Source: three-view drawing plus pictorial views. Frame: mm from the lowest corner of the part. A direction names the side the tool comes from. Round coordinates to 2 decimals unless told otherwise and drop trailing zeros. Write each loop counter-clockwise with the first axis right and the second up, starting at its lowest first coordinate (ties: lowest second). Pieces come first, ordered by that corner, then holes. Notation, with made-up numbers: (70, 0) - (105, 0) arc R25 cw to (105, 35) - close; hole circle Ø10 at (87.25, -20.75). An arc over 180 degrees is marked (long way). Write each question's results on one line, items separated by ' | '.
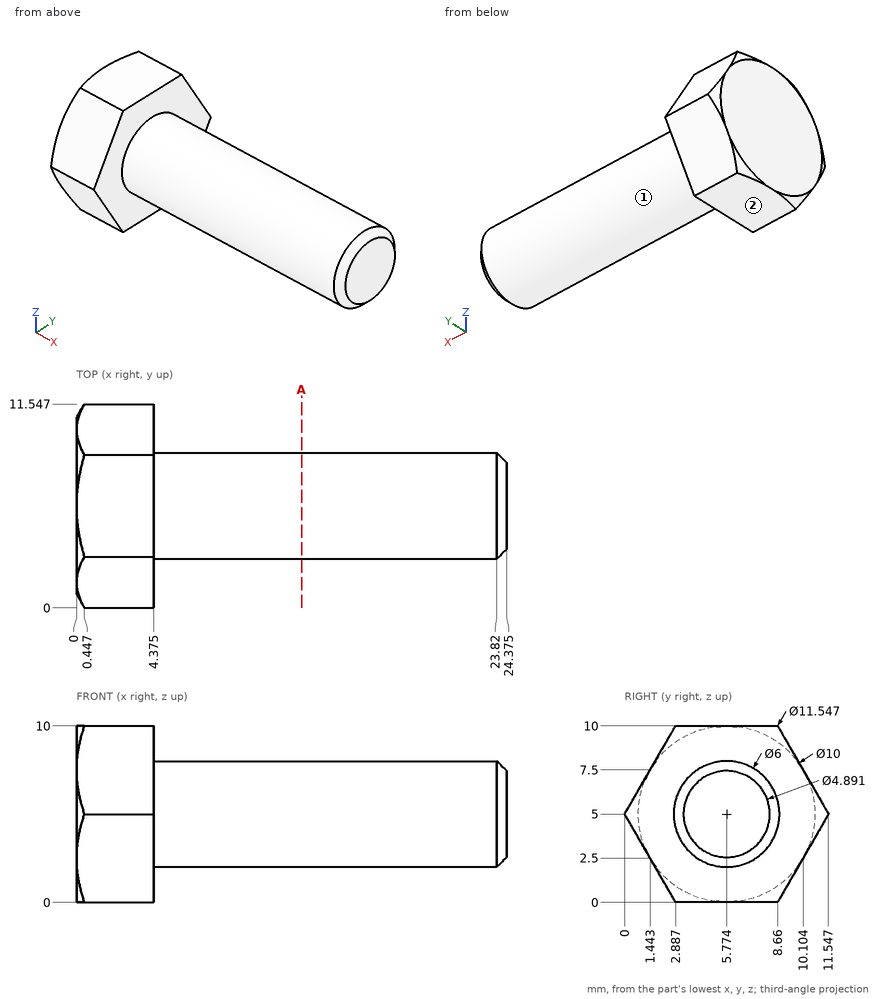
Q1. Access query for the marked faces 1 and 2. Directions: +Z, -Z, +X, -X, +Y, -Y. A direction counts if a zero-diameter tool reaches every point of the face in a straight line with its end or side. Return the directions, or none.
Answer block:
face 1: +X | face 2: -Z, +X, -X, +Y, -Y
Q2. Ray query, line 1 along X through (y, z) = (3, 8.75) (1 decimal); line 2 along Z through (x, y) = (22.5, 3.5) (1 decimal); line 3 along Y through (x, z) = (17, 7) (1 decimal). Return the intervals inside material, ascending.
Answer block:
line 1: 0 to 4.4 | line 2: 3 to 7 | line 3: 3.5 to 8
Q3. Pin query (flat end, axial travel): pin 1 (5 mm diameter, centred on x = 4, z = 2, fed in from -Y); pin 2 (1.5 mm diameter, centred on x = 21.5, z = 2, fed in from -Y); pin 3 (3 mm diameter, centred on x = 14, z = 2.5, fed in from -Y) (1 decimal). Return the tip coordinate at first contact, or that it passes through.
Answer block:
pin 1: y = 0.29 | pin 2: y = 3.79 | pin 3: y = 2.9
Q4. Section query A-A, the plane x = 12.75. Return loops of the section in (y, z).
Answer block:
outline: circle Ø6 at (5.77, 5)
